Geometry: final body of the model. Coordinates: model frame, mm. A direction names the side the tool comes from. Coordinates: 2 decimals unless noted, no trailing zeros. Order: outer loops, then holes, each group sorted by start corner. A loop starts at its lowest first (then second) coordinate and runs counter-clockwise, first axis right, second up. Notation, with made-up numbers: M 24,37.5 L 34,37.5 A11 cw 34,47.5 Z; hole C -19,-20 d4. An arc over 180 degrees is marked long. Use CSV: the item, a comma, the result in double quotes. Start each with the question number.
1. Section query B-B on y = -4.25. Return the cut outline in (x, z).
2. Set-up query: faces 1 (the flat face through (-45.273, -3, 39)), 2 (the flat face through (-68, -3, 11.679)), 3 (the flat face through (-68, -3, -25.321)). Return all of +Z, -Z, +X, -X, +Y, -Y with unobstructed straight access to the full face (end or side cutting, diameter ignored); none if empty.
3. Pull-direction query (X, two-part tool) for faces 4 (the flat face through (-49.821, -3.465, 63.986)), 5 (the flat face through (-43.273, -3, 20)), 6 (the flat face through (-68, -3, 13.679)); classes: pulls with the +X half, pulls with the -X half, needs draft (parallel to the pull), parting line crosses it, or undercut.
4. First-contact query: P1, Ø1.5, axis at x = -75, y = -3, coming from the +Z side; P2, Ø2.5, axis at y = -3, z = 46, coming from the -X side. Flat tips, straight axial feed; report the tip coordinate or a pass-through.
5. Material intervals for line 1 (Z direction, x = -78, y = -4.25); line 2 (X direction, y = -5.5, z = -13); line 3 (X direction, y = -6, z = 24), sorted ascending.
from build123d import *

# Parameters (mm, degrees)
F0_W     = 44
F0_H     = 35
F1_DEPTH = 7
F2_R     = 0.99999


# Not quite as in the source:
# - a fillet or chamfer is up to 0.001 mm smaller than in the source, because OpenCascade refuses the exact size


with BuildPart() as f1:
    # F0 (on Front) → F1 (new body)
    with BuildSketch(Plane.XZ):
        Polygon((-54.2730142517, 66.1785921497), (-54.2730142517, 63.7968573394), (-45.2730142517, 64.1785921497), (-45.2730142517, 13.6785921497), (-91.2730142517, 13.6785921497), (-91.2730142517, 11.6785921497), (-91.2730142517, -23.3214078503), (-91.2730142517, -25.3214078503), (-43.2730142517, -25.3214078503), (-43.2730142517, 66.1785921497), align=None)
        with Locations((-67.2730142517, -5.8214078503)):
            Rectangle(F0_W, F0_H, mode=Mode.SUBTRACT)
    extrude(amount=F1_DEPTH)

    # F2 (radius 1 in the source; OpenCascade refuses exactly that, so slightly less here)
    f2_edges = [f1.edges().sort_by_distance(p)[0] for p in [
        (-48.773014, -7, 66.178592),
        (-54.273014, -7, 64.987725),
        (-49.773014, -7, 63.987725),
        (-45.273014, -7, 38.928592),
        (-68.273014, -7, 13.678592),
        (-91.273014, -7, -5.821408),
        (-67.273014, -7, -25.321408),
        (-43.273014, -7, 20.428592),
        (-45.273014, -7, -5.821408),
        (-67.273014, -7, -23.321408),
        (-89.273014, -7, -5.821408),
        (-67.273014, -7, 11.678592),
        (-48.773014, 0, 66.178592),
        (-54.273014, 0, 64.987725),
        (-49.773014, 0, 63.987725),
        (-45.273014, 0, 38.928592),
        (-68.273014, 0, 13.678592),
        (-91.273014, 0, -5.821408),
        (-67.273014, 0, -25.321408),
        (-43.273014, 0, 20.428592),
        (-45.273014, 0, -5.821408),
        (-67.273014, 0, -23.321408),
        (-89.273014, 0, -5.821408),
        (-67.273014, 0, 11.678592),
        (-45.273014, -3.5, 11.678592),
        (-45.273014, -3.5, -23.321408),
        (-89.273014, -3.5, 11.678592),
        (-89.273014, -3.5, -23.321408),
        (-54.273014, -3.5, 63.796857),
        (-45.273014, -3.5, 64.178592),
        (-54.273014, -3.5, 66.178592),
        (-43.273014, -3.5, 66.178592),
        (-45.273014, -3.5, 13.678592),
        (-43.273014, -3.5, -25.321408),
    ]]
    fillet(f2_edges, radius=F2_R)


solid = f1.part
Results list:
1,outline,"M -91.27,-25.32 L -44.27,-25.32 A1 ccw -43.27,-24.32 L -43.27,65.18 A1 ccw -44.27,66.18 L -53.27,66.18 A1 ccw -54.27,65.18 L -54.27,64.84 A1 ccw -53.23,63.84 L -46.32,64.13 A1 cw -45.27,63.14 L -45.27,14.68 A1 cw -46.27,13.68 L -91.27,13.68 Z; hole M -89.27,-22.32 A1 ccw -88.27,-23.32 L -46.27,-23.32 A1 ccw -45.27,-22.32 L -45.27,10.68 A1 ccw -46.27,11.68 L -88.27,11.68 A1 ccw -89.27,10.68 Z"
2,face 1,"-X, +Y, -Y"
2,face 2,"+Y, -Y"
2,face 3,"-Z, +X, -X, +Y, -Y"
3,face 4,"undercut"
3,face 5,"pulls with the +X half"
3,face 6,"needs draft"
4,P1,"stops at z = 13.68"
4,P2,"stops at x = -45.27"
5,line 1,"z = -25.32 to -23.32, 11.68 to 13.68"
5,line 2,"x = -91.27 to -89.27, -45.27 to -43.27"
5,line 3,"x = -45.27 to -43.27"
